Work out the finished part from the listing and answer in its coordinate system (mm). Coordinates: 2 decimals unless noted, no trailing zeros. Order: outer loops, then holes, each group sorted by start corner. A loop starts at its lowest first (then second) coordinate and runs counter-clockwise, first axis right, second up. Notation, with made-up numbers: M 45,13.25 L 77,13.25 A25 cw 77,29.25 Z; hole C 10.5,47.5 d2. An arc over 180 degrees is marked long. Use a Markdown table: item, result.
from build123d import *

# Parameters (mm, degrees)
BOSS_EXTRUDE1_DEPTH = 16
FILLET6_R           = 8
FILLET7_R           = 8


with BuildPart() as part:
    # Sketch1 → Boss-Extrude1 (new body)
    with BuildSketch(Plane.YZ):
        with BuildLine():
            Line((-27.5, -15), (25.5, -15))
            ThreePointArc((25.5, -15), (26.914213562, -14.414213562), (27.5, -13))
            Line((27.5, -13), (27.5, 13))
            ThreePointArc((27.5, 13), (26.914213562, 14.414213562), (25.5, 15))
            Line((25.5, 15), (-27.5, 15))
            Line((-27.5, 15), (-27.5, -15))
        make_face()
    extrude(amount=BOSS_EXTRUDE1_DEPTH)

    # Fillet6
    # the kernel refuses this fillet: 8 mm, written as the material it takes off along each edge
    with BuildSketch(Plane(origin=(16, 27.5, -33), x_dir=(-1, 0, 0), z_dir=(0, 0, 1))) as fillet6_piece_1:
        with BuildLine():
            CenterArc((FILLET6_R, FILLET6_R), FILLET6_R, 180, 90)
            Line((0, FILLET6_R), (0, 0))
            Line((0, 0), (FILLET6_R, 0))
        make_face()
    extrude(amount=66, mode=Mode.SUBTRACT)

    # Fillet7
    # the kernel refuses this fillet: 8 mm, written as the material it takes off along each edge
    with BuildSketch(Plane(origin=(0, 27.5, -33), x_dir=(0, -1, 0), z_dir=(0, 0, 1))) as fillet7_piece_1:
        with BuildLine():
            CenterArc((FILLET7_R, FILLET7_R), FILLET7_R, 180, 90)
            Line((0, FILLET7_R), (0, 0))
            Line((0, 0), (FILLET7_R, 0))
        make_face()
    extrude(amount=66, mode=Mode.SUBTRACT)


solid = part.part
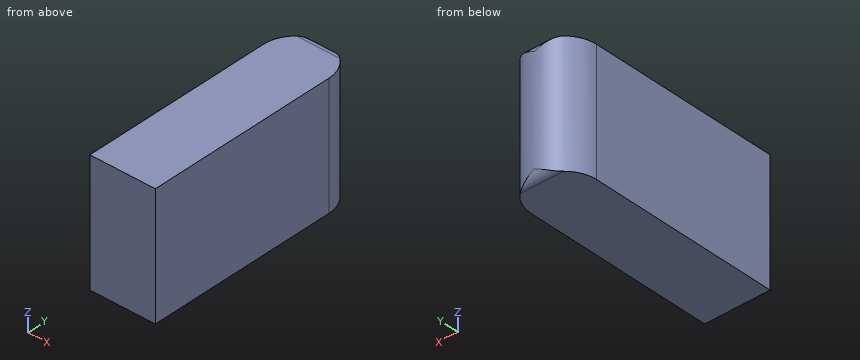
(1) A cutting plane is placed at B-B (x = 2). Determine the outline of the cut face in (y, z).
Conclusion:
| item | result |
|---|---|
| outline | M -27.5,-15 L 24.79,-15 L 24.79,15 L -27.5,15 Z |
(2) Straight lines are drawn through the part: L1, parallel to Y at x = 6.5, z = 1; L2, parallel to Y at x = 15.25, z = -11; L3, parallel to X at y = 23, z = -4.5. For each, find the intervals that lie inside material, in ascending order.
Conclusion:
| item | result |
|---|---|
| L1 | -27.5 to 27.36 |
| L2 | -27.5 to 22.88 |
| L3 | 0.81 to 15.19 |
(3) A cutting plane is placed at A-A (z = -3). Determine the outline of the cut face in (x, y), then the cut area to 3 significant figures.
Conclusion:
| item | result |
|---|---|
| outline | M 0,-27.5 L 16,-27.5 L 16,19.5 A8 ccw 0,19.5 Z |
| area | 853 mm2 |
